For this review, take the finished solid that the model builds, in its own axes (mm). A direction names the side the tool comes from. Give positions to 0.01 mm unless a question says otherwise; leave off trailing zeros. Loops run counter-clockwise (first coordinate to the right, second up) from the corner with the lowest first, then second, coordinate; pieces in that order, holes last. Notation, with made-up numbers: M 80.5,38.5 L 137.5,38.5 A31 cw 137.5,72.5 Z; hole C -40,-1 d6. An arc over 180 degrees is marked long. Use CSV: the item, a comma, the result in double quotes. Start each with the question number.
1. The part is to be moulded in two halves that separate along X. For faces 1 (the face through (-1, 50, 11)), 2 (the face through (60, -1, 11)), 3 (the face through (35.708, -1.352, 16.098)), say which applies: pulls with the +X half, pulls with the -X half, needs draft (parallel to the pull), parting line crosses it, or undercut.
2. Take a section at C-C, the plane z = 19.75. Write out the cut boundary in (x, y) (3 decimals).
3. Insertion check: P1, Ø4.5, axis at x = 40.5, y = 3, coming from the -Z side; P2, Ø12.5, axis at x = 45, y = -35, coming from the +Z side. Each pin has a flat end and moves straight along its axis. Give the tip position at first contact, or say it passes through.
4. Take a section at A-A, the plane y = 0. Write out the cut boundary in (x, z), and give its area (3 significant figures).
5. Take a section at B-B, the plane y = -35. Write out the cut boundary in (x, z) (3 decimals), and give its area (3 significant figures).
6. To check wall thickness, follow line 1 (Y direction, x = 45, z = 20.5) (3 decimals); line 2 (X direction, y = -29, z = 15.5); line 3 (Y direction, x = -48.5, z = 18). State the ranges of each line that lie inside material, in increasing order. Write a range as [from, to].
7. Tool access review of faces 4 (the face through (50.495, 35.242, 6.409)), 5 (the face through (51, 35, 13)), 6 (the face through (32.757, -0.319, 4.437)): name each direction out of +Z, -Z, +X, -X, +Y, -Y from which nothing blocks a thin tool from reaching the whole face with its end or side.
8. Take a section at D-D, the plane y = 33. Write out the cut boundary in (x, z), and give its area (3 significant figures).
from build123d import *

# Parameters (mm, degrees)
F0_W           = 120
F0_H           = 100
F1_DEPTH       = 23
F3_D           = 9
F3_CBORE_D     = 14.5
F3_CBORE_DEPTH = 9
F5_D           = 11
F5_CBORE_D     = 17.25
F5_CBORE_DEPTH = 10


with BuildPart() as f1:
    # F0 (on Top) → F1 (new body)
    with BuildSketch(Plane.XY):
        Rectangle(F0_W, F0_H)
    extrude(amount=F1_DEPTH)

    # F3 (through all)
    with Locations(Plane(origin=(0, 0, 0), x_dir=(1, 0, 0), z_dir=(0, 0, -1))):
        with Locations((-40, 0), (0, 0), (40, 0)):
            CounterBoreHole(F3_D / 2, F3_CBORE_D / 2, F3_CBORE_DEPTH)

    # F5 (through all)
    with Locations(Plane.XY.offset(23)):
        with Locations((-45, 35), (45, 35), (45, -35), (-45, -35)):
            CounterBoreHole(F5_D / 2, F5_CBORE_D / 2, F5_CBORE_DEPTH)


solid = f1.part
Result set:
1,face 1,"needs draft"
1,face 2,"pulls with the +X half"
1,face 3,"undercut"
2,outline,"M -60,-50 L 60,-50 L 60,50 L -60,50 Z; hole C -45,-35 d17.25; hole C -45,35 d17.25; hole C -40,0 d9; hole C 0,0 d9; hole C 40,0 d9; hole C 45,-35 d17.25; hole C 45,35 d17.25"
3,P1,"z = 9"
3,P2,"z = 13"
4,outline,"M -60,0 L -47.25,0 L -47.25,9 L -44.5,9 L -44.5,23 L -60,23 Z; M -35.5,9 L -32.75,9 L -32.75,0 L -7.25,0 L -7.25,9 L -4.5,9 L -4.5,23 L -35.5,23 Z; M 4.5,9 L 7.25,9 L 7.25,0 L 32.75,0 L 32.75,9 L 35.5,9 L 35.5,23 L 4.5,23 Z; M 44.5,9 L 47.25,9 L 47.25,0 L 60,0 L 60,23 L 44.5,23 Z"
4,area,"1,990 mm2"
5,outline,"M -60,0 L -50.5,0 L -50.5,13 L -53.625,13 L -53.625,23 L -60,23 Z; M -39.5,0 L 39.5,0 L 39.5,13 L 36.375,13 L 36.375,23 L -36.375,23 L -36.375,13 L -39.5,13 Z; M 50.5,0 L 60,0 L 60,23 L 53.625,23 L 53.625,13 L 50.5,13 Z"
5,area,"2,130 mm2"
6,line 1,"[-50, -43.625], [-26.375, 26.375], [43.625, 50]"
6,line 2,"[-60, -51.2], [-38.8, 38.8], [51.2, 60]"
6,line 3,"[-50, -42.88], [-27.12, 27.12], [42.88, 50]"
7,face 4,"+Z, -Z"
7,face 5,"+Z"
7,face 6,"-Z"
8,outline,"M -60,0 L -50.12,0 L -50.12,13 L -53.39,13 L -53.39,23 L -60,23 Z; M -39.88,0 L 39.88,0 L 39.88,13 L 36.61,13 L 36.61,23 L -36.61,23 L -36.61,13 L -39.88,13 Z; M 50.12,0 L 60,0 L 60,23 L 53.39,23 L 53.39,13 L 50.12,13 Z"
8,area,"2,160 mm2"
